Design review of the part built by this model. Coordinates are the model's own, in mm. Round coordinates to 2 decimals unless told otherwise and drop trailing zeros. Order: outer loops, then holes, each group sorted by start corner. A loop starts at its lowest first (then second) coordinate and runs counter-clockwise, first axis right, second up. Notation, with made-up numbers: (41, 62.5) - (76, 62.5) arc R29 cw to (76, 89.5) - close; hole circle Ø6 at (-23.5, -35). An arc over 180 degrees is marked (long way). Use CSV: the item, a comma, the result in double quotes. Start each with the question number.
from build123d import *

# Parameters (mm, degrees)
F0_W     = 60.2922588587
F0_H     = 60.7222765684
F1_DEPTH = 50.8
F2_R     = 10.5951307647
F3_DEPTH = 60.7222765684
F4_R     = 5.08
F5_R     = 5.08


with BuildPart() as f1:
    # F0 (on Front) → F1 (new body)
    with BuildSketch(Plane.XZ):
        with Locations((30.1461294293, 30.3611382842)):
            Rectangle(F0_W, F0_H)
    extrude(amount=F1_DEPTH)

    # F2 (on face) → F3 (cut, through all)
    with BuildSketch(Plane.XY.offset(60.7222765684)):
        with Locations((30.1461294293, -25.4)):
            Circle(F2_R)
    extrude(amount=-F3_DEPTH, mode=Mode.SUBTRACT)

    # F4
    f4_edges = [f1.edges().sort_by_distance(p)[0] for p in [
        (60.292259, 0, 30.361138),
    ]]
    fillet(f4_edges, radius=F4_R)

    # F5
    f5_edges = [f1.edges().sort_by_distance(p)[0] for p in [
        (27.606129, 0, 60.722277),
        (27.606129, 0, 0),
        (0, 0, 30.361138),
        (19.550999, -25.4, 60.722277),
        (30.146129, -50.8, 60.722277),
        (0, -25.4, 60.722277),
        (0, -50.8, 30.361138),
        (0, -25.4, 0),
        (60.292259, -27.94, 0),
        (60.292259, -5.08, 30.361138),
        (60.292259, -50.8, 30.361138),
        (60.292259, -27.94, 60.722277),
        (58.804361, -1.487898, 0),
        (30.146129, -50.8, 0),
        (19.550999, -25.4, 0),
    ]]
    fillet(f5_edges, radius=F5_R)


solid = f1.part
Q1. For L1, parallel to X at y = -25, z = 40; L2, parallel to Y at x = 31, z = 17; L3, parallel to Y at x = 29, z = 31.5, list the stretches that pass through material, from the lowest coordinate up. Write a range as [from, to].
Q2. Take a section at A-A (z = 7). State the section outline as (x, y) points.
Q3. Clearance check with a flat-ended pin moving along its axis: pin 1 (12.5 mm diameter, centred on x = 30.15, y = -25.4, fed in from +Z). State where the tip first meets the part, or that it passes through.
Q4. The part is to be moulded in two halves that separate along Y. For faces 1 (the cylindrical face through (40.252, -22.218, 30.715)), 2 (the cylindrical face through (58.844, -49.272, 30.715)), 3 (the flat face through (30, 0, 31)), say which applies: +Y half, -Y half, draft (parallel to the pull), parting line (faces both ways), or undercut.
Q5. Take a section at B-B (y = -25.4). State the section outline as (x, z) points, plus the area to 3 significant figures.
Findings below:
1,L1,"x = [0, 19.56], [40.73, 60.29]"
1,L2,"y = [-50.8, -35.96], [-14.84, 0]"
1,L3,"y = [-50.8, -35.93], [-14.87, 0]"
2,outline,"(0, -45.72) arc R5.08 ccw to (5.08, -50.8) - (55.21, -50.8) arc R5.08 ccw to (60.29, -45.72) - (60.29, -5.08) arc R5.08 ccw to (55.21, 0) - (5.08, 0) arc R5.08 ccw to (0, -5.08) - close; hole circle Ø21.19 at (30.15, -25.4)"
3,pin 1,"passes through"
4,face 1,"undercut"
4,face 2,"-Y half"
4,face 3,"+Y half"
5,outline,"(0, 5.08) arc R5.08 ccw to (5.08, 0) - (14.47, 0) arc R5.08 ccw to (19.55, 5.08) - (19.55, 55.64) arc R5.08 ccw to (14.47, 60.72) - (5.08, 60.72) arc R5.08 ccw to (0, 55.64) - close; (40.74, 5.08) arc R5.08 ccw to (45.82, 0) - (55.21, 0) arc R5.08 ccw to (60.29, 5.08) - (60.29, 55.64) arc R5.08 ccw to (55.21, 60.72) - (45.82, 60.72) arc R5.08 ccw to (40.74, 55.64) - close"
5,area,"2,330 mm^2"
